Build history of the part. All positions in model axes, mm. Coordinates: 2 decimals unless noted, no trailing zeros. Order: outer loops, then holes, each group sorted by start corner. A loop starts at its lowest first (then second) coordinate and runs counter-clockwise, first axis right, second up. Notation, with made-up numbers: (-36.5, 67) - (-20.5, 67) arc R20 cw to (-20.5, 99) - close; hole circle Ø7 at (-39.75, 23.25). An arc over 180 degrees is marked (long way). Write each question's results on one line, items separated by ' | '.
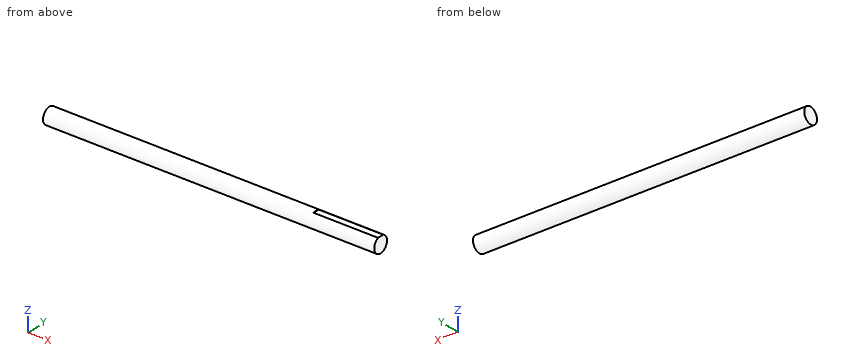
from build123d import *

# Parameters (mm, degrees)
F0_R     = 22.225
F1_DEPTH = 914.4
F3_DEPTH = 177.8
F4_ANGLE = 90


with BuildPart() as f1:
    # F0 (on Right) → F1 (new body)
    with BuildSketch(Plane.YZ):
        Circle(F0_R)
    extrude(amount=F1_DEPTH)

    # F2 (on face) → F3 (cut)
    with BuildSketch(Plane.YZ.offset(914.4)):
        with BuildLine():
            Line((20.3695489641, 8.89), (20.3695489641, -8.89))
            ThreePointArc((20.3695489641, -8.89), (21.7561928049, -4.540781831), (22.225, 0))
            ThreePointArc((22.225, 0), (21.7561928049, 4.540781831), (20.3695489641, 8.89))
        make_face()
    extrude(amount=-F3_DEPTH, mode=Mode.SUBTRACT)


with BuildPart() as f1_1:
    # F4: moved
    add(f1.part.rotate(Axis((0, 0, 0), (1, 0, 0)), F4_ANGLE))


solid = f1_1.part
1. Drop flat-ended pins along their axis: pin 1 Ø3 at (x, z) = (482.5, 12) entering from +Y; pin 2 Ø1.5 at (x, z) = (486, -5.5) entering from -Y; pin 3 Ø3 at (x, z) = (432.5, -2) entering from -Y. Give the stop position or say it passes through.
Solved:
pin 1: stops at y = 19.59 | pin 2: stops at y = -21.71 | pin 3: stops at y = -22.22
2. Band-saw the part on C-C on x = 535.5. Give the cut face in (y, z) (3 decimals), then the cut area to 3 significant figures.
Solved:
outline: circle Ø44.45 at (0, 0) | area: 1,550 mm2
3. Probe line 1 (Z direction, x = 745.5, y = 1.5); line 2 (Z direction, x = 62, y = -2); line 3 (Y direction, x = 323, z = 0) (3 decimals). List the from-to ranges inside material, lowest first.
Solved:
line 1: z = -22.17 to 20.37 | line 2: z = -22.13 to 22.13 | line 3: y = -22.225 to 22.225
4. Band-saw the part on B-B on z = -5. Give the cut face in (x, y).
Solved:
outline: (0, -21.66) - (914.4, -21.66) - (914.4, 21.66) - (0, 21.66) - close
5. Band-saw the part on A-A on x = 816. Give the cut face in (y, z) (3 decimals), then the cut area to 3 significant figures.
Solved:
outline: (-8.89, 20.37) arc R22.225 ccw (long way) to (8.89, 20.37) - close | area: 1,530 mm2
